```python
from build123d import *

# Parameters (mm, degrees)
F0_W     = 7
F0_H     = 53.215195
F0_R     = 1.3
F0_R_2   = 3.81
F0_H_2   = 55.78279
F1_DEPTH = 5.588


with BuildPart() as f1:
    # F0 (on Top) → F1 (new body)
    with BuildSketch(Plane.XY):
        Polygon((41.421356, 100), (-41.421356, 100), (-100, 41.421356), (-100, -41.421356), (-41.421356, -100), (41.421356, -100), (100, -41.421356), (100, 41.421356), align=None)
        Polygon((-63.175, -49.213586), (-63.175, -62.548586), (-70.175, -55.548586), (-70.175, -49.213586), align=None, mode=Mode.SUBTRACT)
        with Locations((-26.67, -62.292402)):
            Rectangle(F0_W, F0_H, mode=Mode.SUBTRACT)
        with Locations((-13.335, -62.292402)):
            Rectangle(F0_W, F0_H, mode=Mode.SUBTRACT)
        with BuildLine():
            ThreePointArc((-63.175, -41.344643), (-62.943305, -42.081527), (-62.865, -42.85))
            ThreePointArc((-62.865, -42.85), (-62.943305, -43.618473), (-63.175, -44.355357))
            ThreePointArc((-63.175, -44.355357), (-70.485, -42.85), (-63.175, -41.344643))
        make_face(mode=Mode.SUBTRACT)
        with Locations((-31.7881, -31.7881)):
            Circle(F0_R, mode=Mode.SUBTRACT)
        with Locations((0, -62.292402)):
            Rectangle(F0_W, F0_H, mode=Mode.SUBTRACT)
        with Locations((13.335, -62.292402)):
            Rectangle(F0_W, F0_H, mode=Mode.SUBTRACT)
        with Locations((26.67, -62.292402)):
            Rectangle(F0_W, F0_H, mode=Mode.SUBTRACT)
        Polygon((70.175, -55.548586), (63.175, -62.548586), (63.175, -49.213586), (70.175, -49.213586), align=None, mode=Mode.SUBTRACT)
        with Locations((31.7881, -31.7881)):
            Circle(F0_R, mode=Mode.SUBTRACT)
        with Locations((66.675, -42.85)):
            Circle(F0_R_2, mode=Mode.SUBTRACT)
        Polygon((49.84, -75.883586), (49.84, 75.883586), (56.84, 68.883586), (56.84, -36.486414), (56.84, -49.213586), (56.84, -68.883586), align=None, mode=Mode.SUBTRACT)
        Polygon((76.51, 49.213586), (83.51, 42.213586), (83.51, -42.213586), (76.51, -49.213586), (76.51, -36.486414), align=None, mode=Mode.SUBTRACT)
        Polygon((-83.51, -42.213586), (-83.51, 42.213586), (-76.51, 49.213586), (-76.51, -36.486414), (-76.51, -49.213586), align=None, mode=Mode.SUBTRACT)
        Polygon((-56.84, -36.486414), (-56.84, 68.883586), (-49.84, 75.883586), (-49.84, -75.883586), (-56.84, -68.883586), (-56.84, -49.213586), align=None, mode=Mode.SUBTRACT)
        Polygon((-70.175, -36.486414), (-70.175, 55.548586), (-63.175, 62.548586), (-63.175, -36.486414), align=None, mode=Mode.SUBTRACT)
        Polygon((-43.505, 82.218586), (-36.505, 88.9), (-36.505, 35.684805), (-36.505, 27.891395), (-36.505, -27.891395), (-36.505, -35.684805), (-36.505, -88.9), (-43.505, -82.218586), align=None, mode=Mode.SUBTRACT)
        with Locations((-26.67, 0)):
            Rectangle(F0_W, F0_H_2, mode=Mode.SUBTRACT)
        with Locations((-13.335, 0)):
            Rectangle(F0_W, F0_H_2, mode=Mode.SUBTRACT)
        with Locations((-31.7881, 31.7881)):
            Circle(F0_R, mode=Mode.SUBTRACT)
        with Locations((-26.67, 62.292402)):
            Rectangle(F0_W, F0_H, mode=Mode.SUBTRACT)
        with Locations((-13.335, 62.292402)):
            Rectangle(F0_W, F0_H, mode=Mode.SUBTRACT)
        Rectangle(F0_W, F0_H_2, mode=Mode.SUBTRACT)
        with Locations((13.335, 0)):
            Rectangle(F0_W, F0_H_2, mode=Mode.SUBTRACT)
        with Locations((26.67, 0)):
            Rectangle(F0_W, F0_H_2, mode=Mode.SUBTRACT)
        Polygon((36.505, 35.684805), (36.505, 88.9), (36.823586, 88.9), (43.505, 82.218586), (43.505, -82.218586), (36.823586, -88.9), (36.505, -88.9), (36.505, -35.684805), (36.505, -27.891395), (36.505, 27.891395), align=None, mode=Mode.SUBTRACT)
        with Locations((31.7881, 31.7881)):
            Circle(F0_R, mode=Mode.SUBTRACT)
        Polygon((63.175, -36.486414), (63.175, 62.548586), (70.175, 55.548586), (70.175, -36.486414), align=None, mode=Mode.SUBTRACT)
        with Locations((0, 62.292402)):
            Rectangle(F0_W, F0_H, mode=Mode.SUBTRACT)
        with Locations((13.335, 62.292402)):
            Rectangle(F0_W, F0_H, mode=Mode.SUBTRACT)
        with Locations((26.67, 62.292402)):
            Rectangle(F0_W, F0_H, mode=Mode.SUBTRACT)
    extrude(amount=F1_DEPTH)


solid = f1.part
```
Geometry: final body of the model. Coordinates: model frame, mm. A direction names the side the tool comes from. Coordinates: 2 decimals unless noted, no trailing zeros. Return JSON: item names as keys, results as strings. Group by question number.
1. Pull-direction query (Y, two-part tool) for faces 3 (the face through (21, 1, 5.588)), 4 (the face through (-56.84, -1, 3)), 5 (the face through (-71.12, -70.3, 2.75)); classes: pulls with the +Y half, pulls with the -Y half, needs draft (parallel to the pull), parting line crosses it, or undercut.
2. Set-up query: faces 1 (the face through (-36.505, 1, 3)), 2 (the face through (70.3, -71.12, 2.75)). Return all of +Z, -Z, +X, -X, +Y, -Y with unobstructed straight access to the full face (end or side cutting, diameter ignored); none if empty.
3. Pin query (flat end, axial travel): pin 1 (1.5 mm diameter, centred on y = 76, z = 1.5, fed in from +X); pin 2 (3 mm diameter, centred on x = -67, z = 4, fed in from +Y); pin 3 (5 mm diameter, centred on x = -42.5, y = -58.5, fed in from +Z); pin 4 (1.7 mm diameter, centred on y = -66, z = 2.5, fed in from -X). Return the tip coordinate at first contact, or that it passes through.
4. Material intervals for line 1 along Y through (x, z) = (-14, 4.6); line 2 along Y through (x, z) = (83, 3.2); line 3 along Y through (x, z) = (-81, 2.95), sorted ascending. Write a range as [from, to].
5. Cut plane A-A (y = -85). Count the separate pieces of the cut face and the enclosed holes in it, plus the area to 3 significant figures.
Resolved:
{
 "1": {"face 3": "needs draft", "face 4": "undercut", "face 5": "pulls with the -Y half"},
 "2": {"face 1": "+Z, -Z", "face 2": "+Z, -Z, +X, -Y"},
 "3": {"pin 1": "stops at x = 66.17", "pin 2": "stops at y = 75.92", "pin 3": "stops at z = 5.59", "pin 4": "stops at x = -76.27"},
 "4": {"line 1": "y = [-100, -88.9], [-35.68, -27.89], [27.89, 35.68], [88.9, 100]", "line 2": "y = [-58.42, -42.72], [42.72, 58.42]", "line 3": "y = [-60.42, -44.72], [44.72, 60.42]"},
 "5": {"separate pieces": "8", "enclosed holes": "0", "area": "389 mm²"}
}
